For this review, take the finished solid that the model builds, in its own axes (mm). A direction names the side the tool comes from. Coordinates: 2 decimals unless noted, no trailing zeros. Loops run counter-clockwise (first coordinate to the right, second up) from the corner with the lowest first, then second, coordinate; pieces in that order, holes last. Notation, with made-up numbers: (-26, -37.5) -> (-17, -37.5) arc R17 ccw to (-17, -21.5) -> close; hole circle Ø4 at (-9, 34.5). An arc over 180 degrees is marked (long way). Answer in a Markdown table with one row per item.
from build123d import *

# Parameters (mm, degrees)
F1_DEPTH       = 50.8
F3_D           = 13.49248
F3_CSINK_D     = 23.8252
F3_CSINK_ANGLE = 82
F4_R           = 6.35
F5_W           = 12.7
F5_H           = 101.6
F6_DEPTH       = 6.35
F7_R           = 12.7
F8_DEPTH       = 101.601


# Not quite as in the source:
# - a feature of the source that left no trace in its solid (it failed there, or was rolled back) is left out


with BuildPart() as f1:
    # F0 (on Front) → F1 (new body, symmetric)
    with BuildSketch(Plane.XZ):
        Polygon((12.601675614, 25.4), (-50.8, 25.4), (-50.8, -25.4), (50.8, -25.4), (50.8, 25.4), align=None)
    extrude(amount=F1_DEPTH, both=True)

    # F3 (through all)
    with Locations(Plane.XY.offset(25.4)):
        with Locations((-31.75, 31.75), (31.75, 31.75), (-31.75, -31.75), (31.75, -31.75)):
            CounterSinkHole(F3_D / 2, F3_CSINK_D / 2, counter_sink_angle=F3_CSINK_ANGLE)

    # F4
    f4_edges = [f1.edges().sort_by_distance(p)[0] for p in [
        (-50.8, 50.8, 0),
        (-50.8, -50.8, 0),
        (50.8, -50.8, 0),
        (50.8, 50.8, 0),
    ]]
    fillet(f4_edges, radius=F4_R)

    # F5 (on face) → F6 (cut)
    with BuildSketch(Plane.XY.offset(25.4)):
        Rectangle(F5_W, F5_H)
    extrude(amount=-F6_DEPTH, mode=Mode.SUBTRACT)

    # F7 (on face) → F8 (cut, through all)
    with BuildSketch(Plane.XZ.offset(50.8)):
        Circle(F7_R)
    extrude(amount=-F8_DEPTH, mode=Mode.SUBTRACT)


solid = f1.part
Item 1: Take a section at D-D, the plane x = -31.75. State the section outline as (y, z) points.
Worked answers:
| item | result |
|---|---|
| outline | (-50.8, -25.4) -> (-38.5, -25.4) -> (-38.5, 19.46) -> (-43.66, 25.4) -> (-50.8, 25.4) -> close; (-25, -25.4) -> (25, -25.4) -> (25, 19.46) -> (19.84, 25.4) -> (-19.84, 25.4) -> (-25, 19.46) -> close; (38.5, -25.4) -> (50.8, -25.4) -> (50.8, 25.4) -> (43.66, 25.4) -> (38.5, 19.46) -> close |
Item 2: The part is to be moulded in two halves that separate along Y. For faces 1 (the flat face through (-11, -50.8, -11)), 2 (the conical face through (-26.197, 27.492, 19.745)), 3 (the flat face through (0, 1, 19.05)), say which applies: +Y half, -Y half, draft (parallel to the pull), parting line (faces both ways), or undercut.
Worked answers:
| item | result |
|---|---|
| face 1 | -Y half |
| face 2 | undercut |
| face 3 | draft |
Item 3: For L1, parallel to X at y = -31.75, z = -14; L2, parallel to Z at x = 0, y = 4.5; L3, parallel to X at y = 7, z = 20, list the stretches that pass through material, from the lowest coordinate up.
Worked answers:
| item | result |
|---|---|
| L1 | -50.8 to -38.5, -25 to 25, 38.5 to 50.8 |
| L2 | -25.4 to -12.7, 12.7 to 19.05 |
| L3 | -50.8 to -6.35, 6.35 to 50.8 |
Item 4: Insertion check: pin 1 (15.5 mm diameter, centred on x = -31.75, y = -31.75, fed in from +Z). The pin has a flat end and moves straight along its axis. Give the tip position at first contact, or say it passes through.
Worked answers:
| item | result |
|---|---|
| pin 1 | z = 20.61 |
Item 5: Take a section at A-A, the plane y = 31.75. State the section outline as (x, z) points.
Worked answers:
| item | result |
|---|---|
| outline | (-50.8, -25.4) -> (-38.5, -25.4) -> (-38.5, 19.46) -> (-43.66, 25.4) -> (-50.8, 25.4) -> close; (-25, -25.4) -> (25, -25.4) -> (25, 19.46) -> (19.84, 25.4) -> (6.35, 25.4) -> (6.35, 19.05) -> (-6.35, 19.05) -> (-6.35, 25.4) -> (-19.84, 25.4) -> (-25, 19.46) -> close; (38.5, -25.4) -> (50.8, -25.4) -> (50.8, 25.4) -> (43.66, 25.4) -> (38.5, 19.46) -> close; hole circle Ø25.4 at (0, 0) |
Item 6: For faces 4 (the cylindrical face through (-2.75, -0.71, -12.4)), 5 (the flat face through (6.35, -1, 22)), list the 3-axis set-ups (+Z, -Z, +X, -X, +Y, -Y) from which the entire face can be reached by the end or side of a thin tool; tool diameter is ignored.
Worked answers:
| item | result |
|---|---|
| face 4 | +Y, -Y |
| face 5 | +Z, +Y, -Y |
Item 7: Take a section at C-C, the plane y = 0. State the section outline as (x, z) points, and give its area (3 significant figures).
Worked answers:
| item | result |
|---|---|
| outline | (-50.8, -25.4) -> (50.8, -25.4) -> (50.8, 25.4) -> (6.35, 25.4) -> (6.35, 19.05) -> (-6.35, 19.05) -> (-6.35, 25.4) -> (-50.8, 25.4) -> close; hole circle Ø25.4 at (0, 0) |
| area | 4,570 mm² |
Item 8: Take a section at B-B, the plane z = 3. State the section outline as (x, y) points.
Worked answers:
| item | result |
|---|---|
| outline | (-50.8, -44.45) arc R6.35 ccw to (-44.45, -50.8) -> (-12.34, -50.8) -> (-12.34, 50.8) -> (-44.45, 50.8) arc R6.35 ccw to (-50.8, 44.45) -> close; (12.34, -50.8) -> (44.45, -50.8) arc R6.35 ccw to (50.8, -44.45) -> (50.8, 44.45) arc R6.35 ccw to (44.45, 50.8) -> (12.34, 50.8) -> close; hole circle Ø13.49 at (-31.75, -31.75); hole circle Ø13.49 at (-31.75, 31.75); hole circle Ø13.49 at (31.75, -31.75); hole circle Ø13.49 at (31.75, 31.75) |
